```python
from build123d import *

# Parameters (mm, degrees)
SKETCH1_W           = 6
SKETCH1_H           = 0.63
BOSS_EXTRUDE1_DEPTH = 6


with BuildPart() as part:
    # Sweep1: sweep along a path in Sketch2
    with BuildLine(Plane.XY) as sweep1_path:
        Line((0, 0), (-342.20186112, 0))
        ThreePointArc((-342.20186112, 0), (-346.778350853, -0.911057943), (-350.657025134, -3.505315192))
        Line((-350.657025134, -3.505315192), (-383.448760524, -36.337742609))
        ThreePointArc((-383.448760524, -36.337742609), (-387.77186112, -38.13), (-392.094961716, -36.337742609))
        Line((-392.094961716, -36.337742609), (-424.886697107, -3.505315192))
        ThreePointArc((-424.886697107, -3.505315192), (-428.765371388, -0.911057943), (-433.34186112, 0))
        Line((-433.34186112, 0), (-1500, 0))
    # Sketch1 → Sweep1 (sweep)
    with BuildSketch(Plane(origin=(0, 0, 0), x_dir=(0, 0, -1), z_dir=(1, 0, 0))):
        with Locations((3, 0.315)):
            Rectangle(SKETCH1_W, SKETCH1_H)
    sweep(path=sweep1_path.line)

    # Sketch3 → Boss-Extrude1 (add, through all)
    with BuildSketch(Plane.XY):
        with BuildLine():
            Line((-1.5, 0.63), (-1.5, 0))
            Line((-1.5, 0), (0, 0))
            Line((0, 0), (0, 0.63))
            ThreePointArc((0, 0.63), (-0.75, 1.38), (-1.5, 0.63))
        make_face()
    extrude(amount=-BOSS_EXTRUDE1_DEPTH)


solid = part.part
```
Check sheet for the modelled part. Datum: model origin and axes. Units: mm. A direction names the side the tool comes from. Give positions to 0.01 mm unless a question says otherwise; leave off trailing zeros. Order: outer loops, then holes, each group sorted by start corner. A loop starts at its lowest first (then second) coordinate and runs counter-clockwise, first axis right, second up. Notation, with made-up numbers: M -32,-28.5 L 27,-28.5 A34 ccw 27,4.5 Z; hole C 34,47.5 d2. An arc over 180 degrees is marked long. Answer in a Markdown table with one row per item.
1) Cross-section at C-C, the plane x = -1258. Enter the section's corners in (y, z), plus the area to 3 significant figures.
Filled sheet:
| item | result |
|---|---|
| outline | M 0,-6 L 0.63,-6 L 0.63,0 L 0,0 Z |
| area | 3.78 mm2 |
2) Cross-section at B-B, the plane z = -5. Enter the section's corners in (x, y).
Filled sheet:
| item | result |
|---|---|
| outline | M -1500,0 L -433.34,0 A11.95 cw -424.89,-3.51 L -392.09,-36.34 A6.11 ccw -383.45,-36.34 L -350.66,-3.51 A11.95 cw -342.2,0 L 0,0 L 0,0.63 A0.75 ccw -1.5,0.63 L -342.2,0.63 A12.58 ccw -351.1,-3.06 L -383.89,-35.89 A5.48 cw -391.65,-35.89 L -424.44,-3.06 A12.58 ccw -433.34,0.63 L -1500,0.63 Z |
3) Thickness scan on L1, parallel to Y at x = -96.5, z = -4.25; L2, parallel to X at y = -6.5, z = -5.25; L3, parallel to X at y = -30.5, z = -2. Record the ranges inside material, lowest first. Write a range as [from, to].
Filled sheet:
| item | result |
|---|---|
| L1 | y = [0, 0.63] |
| L2 | x = [-421.9, -421.01], [-354.54, -353.65] |
| L3 | x = [-397.93, -397.04], [-378.51, -377.62] |
4) Cross-section at A-A, the plane y = -13.5. Enter the section's corners in (x, z).
Filled sheet:
| item | result |
|---|---|
| outline | M -414.9,-6 L -414.01,-6 L -414.01,0 L -414.9,0 Z; M -361.53,-6 L -360.64,-6 L -360.64,0 L -361.53,0 Z |
5) Gauge pin test, flat ends, axial feed: P1, Ø1, axis at y = -11.5, z = -1.5, coming from the +X side; P2, Ø1, axis at x = -168, z = -2, coming from the -Y side; P3, Ø3, axis at x = -136, z = -2, coming from the +Y side. Record the tip position at first contact, or that the pin passes through.
Filled sheet:
| item | result |
|---|---|
| P1 | stops at x = -358.14 |
| P2 | stops at y = 0 |
| P3 | stops at y = 0.63 |
6) Access from +Z, -Z, +X, -X, +Y, -Y to the whole of each face (thin tool, end or side, straight path). Record for faces 1 (the flat face through (-408.72, -19.69, -2.96)), 2 (the flat face through (-367.73, -19.71, -3.04)).
Filled sheet:
| item | result |
|---|---|
| face 1 | +Z, -Z, -X, -Y |
| face 2 | +Z, -Z, +Y |
